The listing builds one solid part. Answer for the finished solid, in the listing's coordinates (mm). A direction names the side the tool comes from. Round coordinates to 2 decimals unless told otherwise and drop trailing zeros. Write each loop counter-clockwise with the first axis right and the second up, starting at its lowest first coordinate (ties: lowest second). Pieces come first, ordered by that corner, then holes.
(1) For faces 1 (the face through (1.73, -7.81, -4.3)), 2 (the face through (-2, -6, -0.5)), 3 (the face through (-5.194, 1.847, -5.766)), determine the directions among +Z, -Z, +X, -X, +Y, -Y from which every point of the face is accessible in a straight line to the end or side of a thin tool.
(2) Each of these flat-tipped pins is pushed along its axis until it touches: pin 1 Ø1.5 at (x, z) = (-3, 2.5) entering from -Y; pin 2 Ø3 at (y, z) = (2, 0.5) entering from -X; pin 3 Ø1.5 at (x, z) = (-4, -4) entering from +Y. Where does it stop, or does it pass through?
(3) The mould has two halves that part along Z. Classify faces 4 (the face through (1.73, -7.81, 7.49)), 5 (the face through (6.094, 0.268, 3.198)), 6 (the face through (-3.4, 0.1, -8)): +Z half, -Z half, draft (parallel to the pull), parting line (faces both ways), or undercut.
(4) A cutting plane is placed at D-D, the plane z = 1.25. Give the vertices of the cut face in (x, y) (3 decimals).
(5) A cutting plane is placed at A-A, the plane y = 0. Give the vertices of the cut face in (x, z) (3 decimals).
(6) A cutting plane is placed at B-B, the plane x = 0. Give the vertices of the cut face in (y, z) (3 decimals), and give its area (3 significant figures).
(7) Find the intervals of material crossed by probe 1 along Y at (x, z) = (0, -2) (3 decimals); probe 2 along Z at (x, y) = (-6.25, 0); probe 3 along Y at (x, z) = (0, 2) (3 decimals), in increasing order.
(8) A cutting plane is placed at C-C, the plane y = 2.5. Give the vertices of the cut face in (x, z), and give its area (3 significant figures).
from build123d import *

# Parameters (mm, degrees)
F2_R     = 3.175
F3_DEPTH = 25
F4_R     = 2
F5_DEPTH = 25


with BuildPart() as f1:
    # F0 (on Front) → F1 (revolve)
    with BuildSketch(Plane.XZ):
        Polygon((-8, -8), (0, -8), (0, 8), (-8, 8), (-8, 7), (-6.1, 7), (-6.1, -0.5), (-8, -0.5), align=None)
    revolve(axis=Axis((0, 0, -0.818246), (0, 0, -1)))

    # F2 (on face) → F3 (cut)
    with BuildSketch(Plane(origin=(0, 0, -8), x_dir=(1, 0, 0), z_dir=(0, 0, -1))):
        Circle(F2_R)
    extrude(amount=-F3_DEPTH, mode=Mode.SUBTRACT)

    # F4 (on Right) → F5 (cut)
    with BuildSketch(Plane.YZ):
        with Locations((0, -5)):
            Circle(F4_R)
    extrude(amount=-F5_DEPTH, mode=Mode.SUBTRACT)


solid = f1.part
Solutions:
1. face 1: +Z, -Z
1. face 2: none
1. face 3: -X
2. pin 1: stops at y = -5.67
2. pin 2: stops at x = -7.95
2. pin 3: stops at y = 7.31
3. face 4: draft
3. face 5: undercut
3. face 6: -Z half
4. outline: circle Ø12.2 at (0, 0); hole circle Ø6.35 at (0, 0)
5. outline: (-8, -8) - (-3.175, -8) - (-3.175, -7) - (-8, -7) - close; (-8, -3) - (-3.175, -3) - (-3.175, 8) - (-8, 8) - (-8, 7) - (-6.1, 7) - (-6.1, -0.5) - (-8, -0.5) - close; (3.175, -8) - (8, -8) - (8, -0.5) - (6.1, -0.5) - (6.1, 7) - (8, 7) - (8, 8) - (3.175, 8) - close
6. outline: (-8, -8) - (-3.175, -8) - (-3.175, 8) - (-8, 8) - (-8, 7) - (-6.1, 7) - (-6.1, -0.5) - (-8, -0.5) - close; (3.175, -8) - (8, -8) - (8, -0.5) - (6.1, -0.5) - (6.1, 7) - (8, 7) - (8, 8) - (3.175, 8) - close
6. area: 126 mm2
7. probe 1: y = -8 to -3.175, 3.175 to 8
7. probe 2: z = -8 to -7, -3 to -0.5, 7 to 8
7. probe 3: y = -6.1 to -3.175, 3.175 to 6.1
8. outline: (-7.6, -8) - (-1.96, -8) - (-1.96, 8) - (-7.6, 8) - (-7.6, 7) - (-5.56, 7) - (-5.56, -0.5) - (-7.6, -0.5) - close; (1.96, -8) - (7.6, -8) - (7.6, -0.5) - (5.56, -0.5) - (5.56, 7) - (7.6, 7) - (7.6, 8) - (1.96, 8) - close
8. area: 150 mm2
